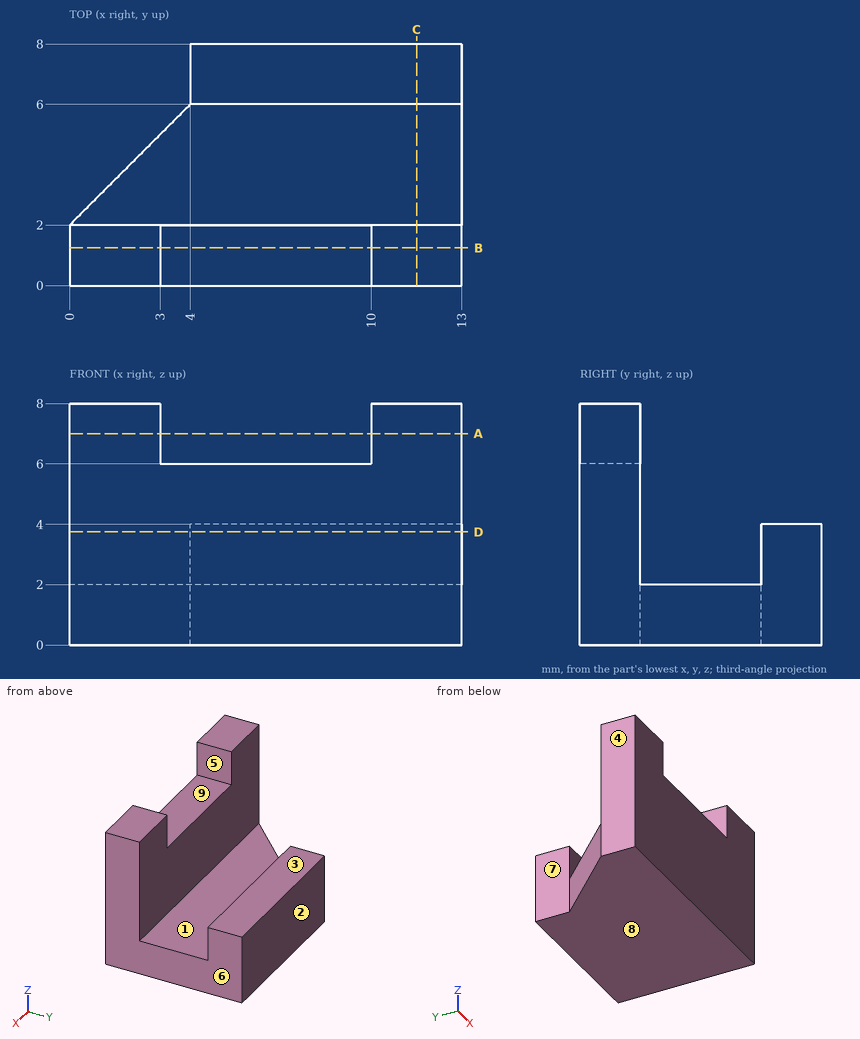
Part print with two shaded views. Sizes in mm from the minimum x, y, z corner. A direction names the side the tool comes from. Round coordinates to 2 decimals unless told otherwise and drop trailing zeros. Write each loop counter-clockwise with the first axis right and the second up, starting at its lowest first coordinate (ties: lowest second). Pieces come first, ordered by that corner, then holes. Notation, with made-up numbers: (46, 2) -> (88, 2) arc R21 cw to (88, 23) -> close; hole circle Ø9 at (15, 83.5). An arc over 180 degrees is marked (long way). Use one line per item in the form item = value.
Q1. Band-saw the part on A-A, the plane z = 7. Write the cut outline in (x, y), then the cut area to 3 significant figures.
Conclusion:
outline = (0, 0) -> (3, 0) -> (3, 2) -> (0, 2) -> close; (10, 0) -> (13, 0) -> (13, 2) -> (10, 2) -> close
area = 12.0 mm²
Q2. Two-plate mould, pull along X, no slides. Class the marked faces 6, 7, 8 and 9: released by +X, released by -X, zero draft, split by the parting line, or undercut.
Conclusion:
face_6 = released by +X
face_7 = released by -X
face_8 = zero draft
face_9 = undercut
Q3. Drill centre lines: L1, parallel to Y at x = 8.75, z = 3.75; L2, parallel to Z at x = 4.5, y = 6.5; L3, parallel to X at y = 7.25, z = 1.75. Where is each one in solid material? Low to high.
Conclusion:
L1 = 0 to 2, 6 to 8
L2 = 0 to 4
L3 = 4 to 13
Q4. Tool access for the marked faces 1, 2, 3, 4 and 5: list every direction of +Z, -Z, +X, -X, +Y, -Y with a clear straight run to the whole face (end or side of a thin tool).
Conclusion:
face_1 = +Z, +X, -X
face_2 = +Z, -Z, +X, -X, +Y
face_3 = +Z, +X, -X, +Y
face_4 = +Z, -Z, -X, +Y, -Y
face_5 = +Z, +Y, -Y
Q5. Band-saw the part on D-D, the plane z = 3.75. Write the cut outline in (x, y), then the cut area to 3 significant figures.
Conclusion:
outline = (0, 0) -> (13, 0) -> (13, 2) -> (0, 2) -> close; (4, 6) -> (13, 6) -> (13, 8) -> (4, 8) -> close
area = 44.0 mm²
Q6. Drop flat-ended pins along their axis: P1, Ø1.6, axis at x = 7, y = 6.5, coming from the +Z side; P2, Ø2, axis at y = 6.5, z = 2.5, coming from the -X side; P3, Ø1.2, axis at x = 8.5, y = 3.5, coming from the +Z side. Give the stop position or say it passes through.
Conclusion:
P1 = 4
P2 = 3.63
P3 = 2
Q7. Band-saw the part on B-B, the plane y = 1.25. Write the cut outline in (x, z).
Conclusion:
outline = (0, 0) -> (13, 0) -> (13, 8) -> (10, 8) -> (10, 6) -> (3, 6) -> (3, 8) -> (0, 8) -> close
Q8. Band-saw the part on C-C, the plane x = 11.5. Write the cut outline in (y, z), then the cut area to 3 significant figures.
Conclusion:
outline = (0, 0) -> (8, 0) -> (8, 4) -> (6, 4) -> (6, 2) -> (2, 2) -> (2, 8) -> (0, 8) -> close
area = 32.0 mm²
